Here's how the part is built. I have some questions about the finished solid (model axes, mm). A direction names the side the tool comes from. Coordinates: 2 decimals unless noted, no trailing zeros. Order: outer loops, then holes, each group sorted by start corner. A loop starts at its lowest first (then second) coordinate and runs counter-clockwise, first axis right, second up. Notation, with made-up numbers: (18.25, 62.25) - (48.25, 62.25) arc R16 cw to (48.25, 71.25) - close; hole circle Ø7 at (55, 8.25). An arc over 180 degrees is marked (long way). Answer in a Markdown table with one row per item. Add a question column.
Item 1: Will these pins go through, and if not, where does the flat tip stop? pin 1 Ø6 at (x, y) = (2, 40) entering from +Z; pin 2 Ø4 at (x, y) = (-5.5, 30) entering from +Z; pin 3 Ø1.1 at (y, z) = (50, 0) entering from -X.
Item 2: I want a section at D-D (y = 25.5). Please give me the cut outline in (x, z), plus the area to 3 significant figures.
Item 3: If I drill on line 1 along Z through (x, y) = (0, 41); line 2 along Y through (x, z) = (2.5, 1); line 3 along Y through (x, z) = (-3, 3), over which ranges is the centre line in solid material (lowest first)? Write a range as from..to.
Item 4: I want a section at B-B (z = 0). Please give me the cut outline in (x, y).
Item 5: On a 3-axis mill with a long thin cutter (end or side, diameter ignored), from which of +Z, -Z, +X, -X, +Y, -Y can I reach the whole of each face in a straight line? I mean faces 1 (the cylindrical face through (-1.5, 46.7, 0)), 2 (the cylindrical face through (0.6, 42, 4.2)), 3 (the flat face through (-1, 51, 0)). Say none if no direction works.
Item 6: I want a section at A-A (y = 43.5). Please give me the cut outline in (x, z).
Item 7: Thinking about a two-plate mould opening in X: for faces 4 (the flat face through (-3.4, 44, -1.7)), 5 (the cylindrical face through (0.6, 42, -5.8)), 6 (the cylindrical face through (3.233, 44.986, -1.341)), which applies, +X half, -X half, draft (parallel to the pull), parting line (faces both ways), or undercut?
Item 8: I want a section at C-C (x = -3). Please give me the cut outline in (y, z).
Autodesk Inventor part; units mm, degrees
ref_plane "YZ Plane" through (0, 0, 0) normal (1, 0, 0) x (0, 1, 0)
ref_plane "XZ Plane" through (0, 0, 0) normal (0, 1, 0) x (-1, 0, 0)
ref_plane "XY Plane" through (0, 0, 0) normal (0, 0, 1) x (1, 0, 0)
sketch "Boceto1" plane through (0, 0, 0) normal (0, 1, 0) x (-1, 0, 0)
  circle A0 centre (0, 0) radius 8
  dimension "d0" = 16
extrude "Extrusión1" add sketch "Boceto1" along normal blind 44
sketch "Boceto2" plane through (0, 44, 0) normal (0, 1, 0) x (1, 0, 0)
  circle A0 centre (0, 0) radius 3.5
  dimension "d3" = 7
extrude "Extrusión2" add sketch "Boceto2" along normal blind 2
sketch "Boceto3" plane through (0, 46, 0) normal (0, 1, 0) x (1, 0, 0)
  arc A0 (-1, -1.118) -> (-1, 1.118) centre (0, 0) ccw
  line L0 (1.5, 0) -> (-1, 0)
  line L1 (-1, 0) -> (-1, 1.118)
  line L2 (-1, 0) -> (-1, -1.118)
  dimension "d6" = 3
  dimension "d7" = 2.5
extrude "Extrusión3" add sketch "Boceto3" along normal blind 7.8
sketch "Boceto4" plane through (0, 46, 0) normal (0, 1, 0) x (1, 0, 0)
  line L0 (-1, 1.118) -> (-1, -1.118)
  circle A0 centre (0, 0) radius 1.5
extrude "Extrusión4" add sketch "Boceto4" along normal blind 1.5 contours L0 A0 picked at (-1.1631, -0.0599)
sketch "Boceto5" plane through (0, 44, 0) normal (0, 1, 0) x (1, 0, 0)
  circle A0 centre (0, 0) radius 1.5
  circle A1 centre (0, 0) radius 5
  circle A2 centre (0, 5) radius 1
  circle A3 centre (0, -5) radius 1
  dimension "d12" = 10
  dimension "d13" = 2
  dimension "d14" = 2
hole "Agujero1" at (0, 44, -5) at (0, 44, 5) direction (0, -1, 0) diameter 2 depth 4 tip angle 118
properties part number "motor2"
Values follow:
| question | item | result |
|---|---|---|
| 1 | pin 1 | stops at z = 8 |
| 1 | pin 2 | stops at z = 7.19 |
| 1 | pin 3 | stops at x = -1 |
| 2 | outline | circle Ø16 at (0, 0) |
| 2 | area | 201 mm^2 |
| 3 | line 1 | z = -8..-6, -4..4, 6..8 |
| 3 | line 2 | y = 0..46 |
| 3 | line 3 | y = 0..44 |
| 4 | outline | (-8, 0) - (8, 0) - (8, 44) - (3.5, 44) - (3.5, 46) - (1.5, 46) - (1.5, 53.8) - (-1, 53.8) - (-1, 47.5) - (-1.5, 47.5) - (-1.5, 46) - (-3.5, 46) - (-3.5, 44) - (-8, 44) - close |
| 5 | face 1 | -X, +Y |
| 5 | face 2 | +Y |
| 5 | face 3 | +Z, -Z, -X, +Y |
| 6 | outline | circle Ø16 at (0, 0); hole circle Ø2 at (0, -5); hole circle Ø2 at (0, 5) |
| 7 | face 4 | draft |
| 7 | face 5 | undercut |
| 7 | face 6 | parting line |
| 8 | outline | (0, -7.42) - (44, -7.42) - (44, -1.8) - (46, -1.8) - (46, 1.8) - (44, 1.8) - (44, 7.42) - (0, 7.42) - close |
